from build123d import *

# Parameters (mm, degrees)
SKETCH1_R               = 38.227
BOSS_EXTRUDE1_DEPTH     = 142.8496
SKETCH2_R               = 2.413
CUT_EXTRUDE1_DEPTH      = 143.8496
SKETCH3_R               = 12.1285
CUT_EXTRUDE2_DEPTH      = 143.8496
SKETCH4_R               = 3.175
CUT_EXTRUDE3_DEPTH      = 6.35
SKETCH5_R               = 10.16
CUT_EXTRUDE4_DEPTH      = 17.78
SKETCH6_R               = 2.38125
CUT_EXTRUDE5_DEPTH      = 1
CUT_EXTRUDE5_DEPTH_BACK = 143.8496


with BuildPart() as part:
    # Sketch1 → Boss-Extrude1 (new body)
    with BuildSketch(Plane(origin=(0, 0, 0), x_dir=(1, 0, 0), z_dir=(0, 1, 0))):
        Circle(SKETCH1_R)
    extrude(amount=BOSS_EXTRUDE1_DEPTH)

    # Sketch2 → Cut-Extrude1 (cut, through all)
    with BuildSketch(Plane(origin=(0, 142.8496, 0), x_dir=(1, 0, 0), z_dir=(0, 1, 0))):
        with Locations((0, 29.337)):
            Circle(SKETCH2_R)
        with Locations((25.406587271, -14.6685)):
            Circle(SKETCH2_R)
        with Locations((-25.406587271, -14.6685)):
            Circle(SKETCH2_R)
    extrude(amount=-CUT_EXTRUDE1_DEPTH, mode=Mode.SUBTRACT)

    # Sketch3 → Cut-Extrude2 (cut, through all)
    with BuildSketch(Plane(origin=(0, 142.8496, 0), x_dir=(1, 0, 0), z_dir=(0, 1, 0))):
        with Locations((-12.7, 10.16)):
            Circle(SKETCH3_R)
        with Locations((12.7, 10.16)):
            Circle(SKETCH3_R)
    extrude(amount=-CUT_EXTRUDE2_DEPTH, mode=Mode.SUBTRACT)

    # Sketch4 → Cut-Extrude3 (cut)
    with BuildSketch(Plane(origin=(0, 142.8496, 0), x_dir=(1, 0, 0), z_dir=(0, 1, 0))):
        with Locations((0, 20.32)):
            Circle(SKETCH4_R)
        Circle(SKETCH4_R)
    extrude(amount=-CUT_EXTRUDE3_DEPTH, mode=Mode.SUBTRACT)

    # Sketch5 → Cut-Extrude4 (cut)
    with BuildSketch(Plane(origin=(0, 142.8496, 0), x_dir=(1, 0, 0), z_dir=(0, 1, 0))):
        with Locations((0, -18.415)):
            Circle(SKETCH5_R)
    extrude(amount=-CUT_EXTRUDE4_DEPTH, mode=Mode.SUBTRACT)

    # Sketch6 → Cut-Extrude5 (cut, two sides)
    with BuildSketch(Plane(origin=(0, 142.8496, 0), x_dir=(1, 0, 0), z_dir=(0, 1, 0))) as cut_extrude5_sk:
        with Locations((15.875, -10.16)):
            Circle(SKETCH6_R)
    extrude(amount=CUT_EXTRUDE5_DEPTH, mode=Mode.SUBTRACT)
    extrude(cut_extrude5_sk.sketch, amount=-CUT_EXTRUDE5_DEPTH_BACK, mode=Mode.SUBTRACT)


solid = part.part
Work out the finished part from the listing and answer in its coordinate system (mm). A direction names the side the tool comes from. Coordinates: 2 decimals unless noted, no trailing zeros. Loops run counter-clockwise (first coordinate to the right, second up) from the corner with the lowest first, then second, coordinate; pieces in that order, holes last. Notation, with made-up numbers: (21.25, 8) -> (32.25, 8) arc R20 cw to (32.25, 24) -> close; hole circle Ø4 at (-4, -13). An arc over 180 degrees is marked (long way). Write each question's results on one line, items separated by ' | '. Start each with the question number.
1) The mould has two halves that part along Z. Classify faces 1 (the flat face through (-1, 0, -1)), 2 (the cylindrical face through (-28.17, 70.42, -25.84)), 3 (the cylindrical face through (-25.93, 72.425, 17.024)): pulls with the +Z half, pulls with the -Z half, needs draft (parallel to the pull), parting line crosses it, or undercut.
2) Find section D-D on x = -12.7. Determine the outline of the cut face in (y, z), then the cut area to 3 significant figures.
3) Find section B-B on y = 81. Determine the outline of the cut face in (x, z) (1 decimal), then the cut area to 3 significant figures.
4) Find section A-A on z = 0. Determine the outline of the cut face in (x, y) (3 decimals).
5) Find section C-C on z = 10.16. Determine the outline of the cut face in (x, y).
6) Consider line 1 along Z through (x, y) = (0, 138.5) (3 decimals); line 2 along Z through (x, y) = (0, 134.75) (3 decimals); line 3 along Z through (x, y) = (0, 34.5). Determine where each line is inside the solid, lowest interval first.
7) For faces 4 (the cylindrical face through (-0.69, 139.72, 3.1)), 5 (the cylindrical face through (18.146, 72.425, 9.445)), determine the directions among +Z, -Z, +X, -X, +Y, -Y from which every point of the face is accessible in a straight line to the end or side of a thin tool.
8) Flat-ended cylindrical pins translate along their axes: P1, Ø14.5, axis at x = 12.7, z = -10.16, coming from the -Y side; P2, Ø8, axis at y = 114, z = -29, coming from the -X side; P3, Ø10, axis at x = -11.5, y = 41.5, coming from the -Z side; P4, Ø16.5, axis at x = 0, z = 18.415, coming from the +Y side. Find the tip coordinate at first contact, or state that the pin passes through.
Response values:
1) face 1: needs draft | face 2: parting line crosses it | face 3: undercut
2) outline: (0, -36.06) -> (142.85, -36.06) -> (142.85, -22.29) -> (0, -22.29) -> close; (0, 1.97) -> (142.85, 1.97) -> (142.85, 36.06) -> (0, 36.06) -> close | area: 6,840 mm^2
3) outline: circle Ø76.5 at (0, 0); hole circle Ø4.8 at (-25.4, 14.7); hole circle Ø24.3 at (-12.7, -10.2); hole circle Ø4.8 at (0, -29.3); hole circle Ø24.3 at (12.7, -10.2); hole circle Ø4.8 at (15.9, 10.2); hole circle Ø4.8 at (25.4, 14.7) | area: 3,590 mm^2
4) outline: (-38.227, 0) -> (-19.324, 0) -> (-19.324, 142.85) -> (-38.227, 142.85) -> close; (-6.076, 0) -> (6.076, 0) -> (6.076, 142.85) -> (3.175, 142.85) -> (3.175, 136.5) -> (-3.175, 136.5) -> (-3.175, 142.85) -> (-6.076, 142.85) -> close; (19.324, 0) -> (38.227, 0) -> (38.227, 142.85) -> (19.324, 142.85) -> close
5) outline: (-36.85, 0) -> (13.49, 0) -> (13.49, 142.85) -> (5.92, 142.85) -> (5.92, 125.07) -> (-5.92, 125.07) -> (-5.92, 142.85) -> (-36.85, 142.85) -> close; (18.26, 0) -> (36.85, 0) -> (36.85, 142.85) -> (18.26, 142.85) -> close
6) line 1: z = -38.227 to -31.75, -26.924 to -23.495, -17.145 to -3.175, 3.175 to 8.255, 28.575 to 38.227 | line 2: z = -38.227 to -31.75, -26.924 to 8.255, 28.575 to 38.227 | line 3: z = -38.23 to -31.75, -26.92 to 38.23
7) face 4: +Y | face 5: +Y, -Y
8) P1: passes through | P2: stops at x = -28.92 | P3: stops at z = -37.67 | P4: stops at y = 125.07
